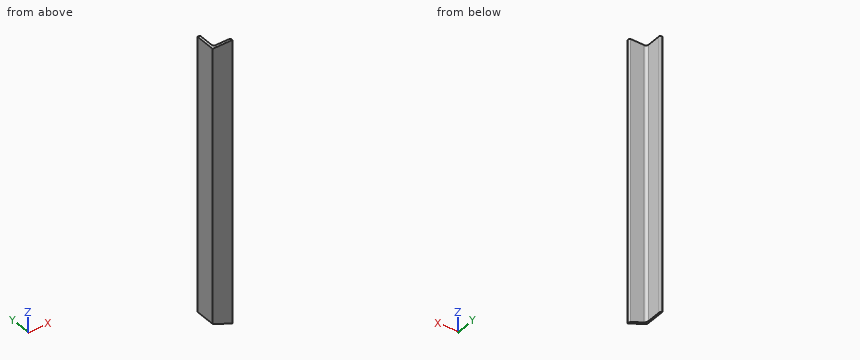
Autodesk Inventor part; units mm, degrees
ref_plane "Start Plane" through (0, 0, 16.9391) normal (0, 0, 1) x (1, 0, 0)
ref_plane "End Plane" through (0, 0, 375.3926) normal (0, 0, 1) x (1, 0, 0)
ref_plane "Work Plane5" through (690, 0.6642, 374.7455) normal (0, -0.0261508, 0.999658) x (1, 0, 0)
ref_plane "Start Plane" through (0, 0, 16.9391) normal (0, 0, 1) x (1, 0, 0)
ref_plane "End Plane" through (0, 0, 375.3926) normal (0, 0, 1) x (1, 0, 0)
sketch "Sketch" plane through (0, 0, 0) normal (0, 0, 1) x (1, 0, 0)
  line L0 (25.4, 0) -> (0, 0)
  line L1 (0, 0) -> (0, 25.4)
  line L2 (0, 25.4) -> (1.651, 25.4)
  line L3 (3.175, 23.876) -> (3.175, 6.477)
  line L4 (6.477, 3.175) -> (23.876, 3.175)
  line L5 (25.4, 1.651) -> (25.4, 0)
  line L6 (0, -11.0414) -> (0, 31.5385) construction
  line L7 (-11.0414, 0) -> (31.5385, 0) construction
  arc A0 (3.175, 6.477) -> (6.477, 3.175) centre (6.477, 6.477) ccw
  arc A1 (3.175, 23.876) -> (1.651, 25.4) centre (1.651, 23.876) ccw
  arc A2 (25.4, 1.651) -> (23.876, 3.175) centre (23.876, 1.651) ccw
  line L8 (0, 40.0545) -> (0, -19.5574) construction
  line L9 (-19.5574, 0) -> (40.0545, 0) construction
  point P0 (3.175, 25.4)
  point P1 (3.175, 3.175)
  point P2 (25.4, 3.175)
  dimension "d0" = 25.4
  dimension "d1" = 25.4
  dimension "d2" = 3.175
  dimension "d3" = 3.175
  dimension "d10" = 0
  dimension "d11" = 0
  dimension "d14" = 3.302
  dimension "d15" = 1.524
extrude "Body" add sketch "Sketch" along normal up to surface (358.4535 mm away) from surface at 16.9391
sketch "Sketch3" plane through (0, 0, 0) normal (0, 0, 1) x (1, 0, 0)
  line L0 (0, 0) -> (10, 0)
ref_plane "Work Plane3" through (0, 0, 0) normal (0, -1, 0) x (1, 0, 0)
ref_plane "Work Plane5" through (690, 0.6642, 374.7455) normal (0, -0.0261508, 0.999658) x (1, 0, 0)
split "Split2" plane through (690, 0.6642, 374.7455) removes the side toward (0, -0.0261508, 0.999658)
ref_plane "Work Plane6" through (249.7692, 1061.6394, -48.8078) normal (-0.3846154, 0.0241392, -0.9227612) x (-0.9152171, 0.1202029, 0.3846154)
split "Split3" plane through (249.7692, 1061.6394, -48.8078) removes the side toward (-0.3846154, 0.0241392, -0.9227612)
sketch "Sketch4" plane through (0, 0, 0) normal (0, -1, 0) x (1, 0, 0)
  line L0 (-2, 16.9391) -> (12, 16.9391)
  line L1 (-2, 375.3926) -> (12, 375.3926)
  dimension "d17" = 358.4535
equation "\"d0\" = G_H"
equation "\"d1\" = G_H"
equation "\"d2\" = G_T"
equation "\"d3\" = G_T"
equation "\"d14\" = G_IR"
equation "\"d15\" = G_ER"
equation "\"d4\" = G_L"
equation "\"G_H\" = 25.4"
equation "\"G_T\" = 3.175"
equation "\"G_ER\" = 1.524"
equation "\"G_IR\" = 3.302"
equation "\"G_L\" = d17"
equation "\"ex\" = 0"
equation "\"G_OFFSET_START\" = -16.93913"
equation "\"G_OFFSET_END\" = -24.74423"
equation "\"d12\" = -G_OFFSET_START"
equation "\"d13\" = G_OFFSET_END + B_L"
equation "\"B_L\" = 400.13684"
properties part number "AISC - L 1 x 1 x 1/8 - 14.112" material "Steel, Mild"
For this review, take the finished solid that the model builds, in its own axes (mm). Give positions to 0.01 mm unless a question says otherwise; leave off trailing zeros. Write each loop counter-clockwise with the first axis right and the second up, starting at its lowest first coordinate (ties: lowest second). Pieces come first, ordered by that corner, then holes. Notation, with made-up numbers: M 33,-35 L 74,-35 A21 ccw 74,-6 Z; hole C 86,-33 d1. An arc over 180 degrees is marked long. One line per item, written item: value.
1) For P1, Ø3, axis at y = 7, z = 249, coming from the +X side; P2, Ø6, axis at y = 17.5, z = 163, coming from the +X side (3 decimals); P3, Ø12, axis at x = 14, z = 304, coming from the +Y side (3 decimals); P4, Ø10, axis at y = 6, z = 190, coming from the +X side, all flat-tipped, find the tip position at first contact; note any pin that passes through.
Results are:
P1: stops at x = 3.32
P2: stops at x = 3.175
P3: stops at y = 3.175
P4: stops at x = 25.4
2) Take a section at B-B, the plane x = 18.5. Write out the cut boundary in (y, z) (3 decimals).
Results are:
outline: M 0,19.815 L 3.175,19.898 L 3.175,374.811 L 0,374.728 Z
3) Take a section at C-C, the plane y = 15. Write out the cut boundary in (x, z) (3 decimals), then the cut area to 3 significant figures.
Results are:
outline: M 0,27.918 L 3.175,26.595 L 3.175,375.121 L 0,375.121 Z
area: 1,100 mm²
4) Take a section at A-A, the plane z = 298.5. Write out the cut boundary in (x, y) (3 decimals).
Results are:
outline: M 0,0 L 25.4,0 L 25.4,1.651 A1.524 ccw 23.876,3.175 L 6.477,3.175 A3.302 cw 3.175,6.477 L 3.175,23.876 A1.524 ccw 1.651,25.4 L 0,25.4 Z
5) For line 1 (X direction, y = 17, z = 141.5) (3 decimals); line 2 (X direction, y = 4.75, z = 143), list the stretches that pass through material, from the lowest coordinate up. Write a range as from..to.
Results are:
line 1: x = 0..3.175
line 2: x = 0..3.66
